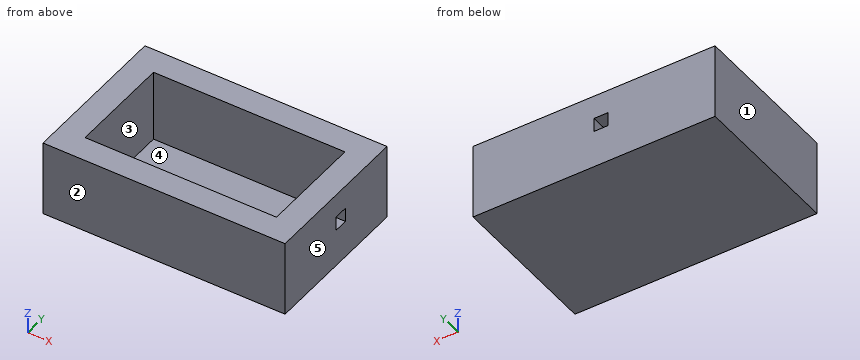
```python
from build123d import *

# Parameters (mm, degrees)
F0_W      = 48
F0_H      = 26
F1_DEPTH  = 1
F0_H_2    = 1.2748
F0_W_2    = 1.273
F2_DEPTH  = 19
F4_W      = 50.546
F4_H      = 19
F4_W_2    = 3.4925
F4_H_2    = 3.4925
F5_DEPTH  = 5.08
F3_W      = 50.546
F3_H      = 19
F6_DEPTH  = 5.08
F7_W      = 38.7096
F7_H      = 19
F7_W_2    = 3.556
F7_H_2    = 3.556
F9_DEPTH  = 5.08
F8_W      = 38.7096
F8_H      = 19
F10_DEPTH = 5.08


with BuildPart() as f1:
    # F0 (on Top) → F1 (new body)
    with BuildSketch(Plane.XY):
        Rectangle(F0_W, F0_H)
    extrude(amount=F1_DEPTH)

    # F0 (on Top) → F2 (join)
    with BuildSketch(Plane.XY):
        with Locations((0, -13.6374)):
            Rectangle(F0_W, F0_H_2)
        with Locations((0, 13.6374)):
            Rectangle(F0_W, F0_H_2)
        with Locations((24.6365, 0)):
            Rectangle(F0_W_2, F0_H)
        with Locations((-24.6365, 0)):
            Rectangle(F0_W_2, F0_H)
        with Locations((-24.6365, -13.6374)):
            Rectangle(F0_W_2, F0_H_2)
        with Locations((24.6365, -13.6374)):
            Rectangle(F0_W_2, F0_H_2)
        with Locations((24.6365, 13.6374)):
            Rectangle(F0_W_2, F0_H_2)
        with Locations((-24.6365, 13.6374)):
            Rectangle(F0_W_2, F0_H_2)
    extrude(amount=F2_DEPTH)

    # F4 (on face) → F5 (join)
    with BuildSketch(Plane(origin=(0, 14.2748, 0), x_dir=(-1, 0, 0), z_dir=(0, 1, 0))):
        with Locations((0, 9.5)):
            Rectangle(F4_W, F4_H)
        with Locations((1.74625, 11.24625)):
            Rectangle(F4_W_2, F4_H_2, mode=Mode.SUBTRACT)
    extrude(amount=F5_DEPTH)

    # F3 (on face) → F6 (join)
    with BuildSketch(Plane.XZ.offset(14.2748)):
        with Locations((0, 9.5)):
            Rectangle(F3_W, F3_H)
    extrude(amount=F6_DEPTH)

    # F7 (on face) → F9 (join)
    with BuildSketch(Plane.YZ.offset(25.273)):
        with Locations((0, 9.5)):
            Rectangle(F7_W, F7_H)
        with Locations((1.778, 11.278)):
            Rectangle(F7_W_2, F7_H_2, mode=Mode.SUBTRACT)
    extrude(amount=F9_DEPTH)

    # F8 (on face) → F10 (join)
    with BuildSketch(Plane(origin=(-25.273, 0, 0), x_dir=(0, -1, 0), z_dir=(-1, 0, 0))):
        with Locations((0, 9.5)):
            Rectangle(F8_W, F8_H)
    extrude(amount=F10_DEPTH)


solid = f1.part
```
For this review, take the finished solid that the model builds, in its own axes (mm). Face numbers are marked on the shaded views. A direction names the side the tool comes from. Coordinates: 2 decimals unless noted, no trailing zeros. Write each loop counter-clockwise with the first axis right and the second up, starting at its lowest first coordinate (ties: lowest second). Pieces come first, ordered by that corner, then holes.
(1) Add section A-A on z = 17.75. Give the boundary of the cut face in (x, y), then the cut area to 3 significant figures.
(2) The part is to be moulded in two halves that separate along X. For the marked faces 1, 2 and 3, say which applies: +X half, -X half, draft (parallel to the pull), parting line (faces both ways), or undercut.
(3) Add section C-C on y = 1. Give the boundary of the cut face in (x, z), then the cut area to 3 significant figures.
(4) Add section B-B on x = 17.5. Give the boundary of the cut face in (y, z).
(5) Wall thickness on probe 1 along X at (y, z) = (5, 13.25); probe 2 along X at (y, z) = (17, 10.5); probe 3 along Y at (x, z) = (-18.5, 17.5): over which ranges is each line inside the solid? List them lowest first.
(6) Add section D-D on x = -2. Give the boundary of the cut face in (y, z).
(7) For pin 1 Ø2 at (x, y) = (15.5, -2.5) entering from +Z, flat-tipped, find the tip position at first contact; note if it passes through.
(8) Tool access review of the marked faces 4 and 5: name each direction out of +Z, -Z, +X, -X, +Y, -Y from which nothing blocks a thin tool from reaching the whole face with its end or side.
Answer sheet:
1. outline: (-30.35, -19.35) - (30.35, -19.35) - (30.35, 19.35) - (-30.35, 19.35) - close; hole (-24, -13) - (24, -13) - (24, 13) - (-24, 13) - close
1. area: 1,100 mm2
2. face 1: -X half
2. face 2: draft
2. face 3: undercut
3. outline: (-30.35, 0) - (30.35, 0) - (30.35, 9.5) - (25.27, 9.5) - (25.27, 13.06) - (30.35, 13.06) - (30.35, 19) - (24, 19) - (24, 1) - (-24, 1) - (-24, 19) - (-30.35, 19) - close
3. area: 271 mm2
4. outline: (-19.35, 0) - (19.35, 0) - (19.35, 19) - (13, 19) - (13, 1) - (-13, 1) - (-13, 19) - (-19.35, 19) - close
5. probe 1: x = -30.35 to -24, 24 to 30.35
5. probe 2: x = -30.35 to -3.49, 0 to 30.35
5. probe 3: y = -19.35 to -13, 13 to 19.35
6. outline: (-19.35, 0) - (19.35, 0) - (19.35, 9.5) - (14.27, 9.5) - (14.27, 12.99) - (19.35, 12.99) - (19.35, 19) - (13, 19) - (13, 1) - (-13, 1) - (-13, 19) - (-19.35, 19) - close
7. pin 1: stops at z = 1
8. face 4: +Z
8. face 5: +Z, -Z, +X, +Y, -Y
